Answer from the drawing. Dimensions are ordinates in mm from the lowest x, y and z of the part. A direction names the side the tool comes from. Give positions to 0.01 mm unless a question says otherwise; leave off trailing zeros. Loops run counter-clockwise (first coordinate to the right, second up) from the corner with the lowest first, then second, coordinate; pieces in that order, holes last. Notation, with made-up numbers: M 44,25.25 L 86,25.25 A22 cw 86,43.25 Z; hole C 65,70 d10. An arc over 180 degrees is marked long. Return JSON: item names as keys, results as strings. Group by question number.
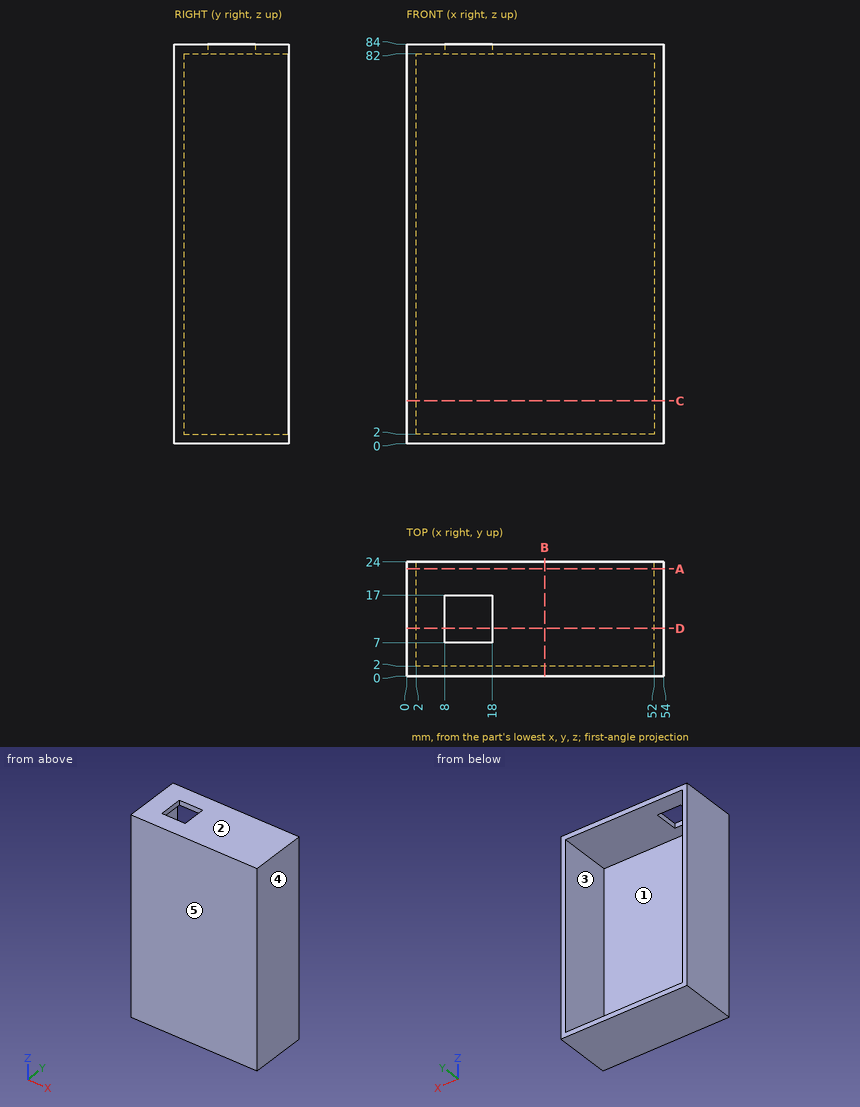
1. A flat-ended cylindrical pin translates along its axis: P1, Ø4, axis at x = 30.5, z = 26, coming from the +Y side. Find the tip coordinate at first contact, or state that the pin passes through.
2. The mould has two halves that part along X. Classify the marked faces 3, 4 and 5: +X half, -X half, draft (parallel to the pull), parting line (faces both ways), or undercut.
3. Find section A-A (y = 22.5). Write down the section's boundary in (x, z), and give its area (3 significant figures).
4. For the marked faces 1 and 2, determine the directions among +Z, -Z, +X, -X, +Y, -Y from which every point of the face is accessible in a straight line to the end or side of a thin tool.
5. Find section D-D (y = 10). Write down the section's boundary in (x, z).
6. Straight lines are drawn through the part: line 1 along X through (y, z) = (23.25, 25); line 2 along Z through (x, y) = (34, 11.5); line 3 along Y through (x, z) = (22.5, 22.5). For each, find the intervals that lie inside material, in ascending order.
7. Find section C-C (z = 9). Write down the section's boundary in (x, y).
8. Find section B-B (x = 29). Write down the section's boundary in (y, z), and give its area (3 significant figures).
Result:
{
 "1": {"P1": "stops at y = 2"},
 "2": {"face 3": "undercut", "face 4": "+X half", "face 5": "draft"},
 "3": {"outline": "M 0,0 L 54,0 L 54,84 L 0,84 Z; hole M 2,2 L 52,2 L 52,82 L 2,82 Z", "area": "536 mm2"},
 "4": {"face 1": "+Y", "face 2": "+Z, +X, -X, +Y, -Y"},
 "5": {"outline": "M 0,0 L 54,0 L 54,84 L 18,84 L 18,82 L 52,82 L 52,2 L 2,2 L 2,82 L 8,82 L 8,84 L 0,84 Z"},
 "6": {"line 1": "x = 0 to 2, 52 to 54", "line 2": "z = 0 to 2, 82 to 84", "line 3": "y = 0 to 2"},
 "7": {"outline": "M 0,0 L 54,0 L 54,24 L 52,24 L 52,2 L 2,2 L 2,24 L 0,24 Z"},
 "8": {"outline": "M 0,0 L 24,0 L 24,2 L 2,2 L 2,82 L 24,82 L 24,84 L 0,84 Z", "area": "256 mm2"}
}
